Work out the finished part from the listing and answer in its coordinate system (mm). A direction names the side the tool comes from. Give positions to 0.01 mm unless a question says otherwise; leave off trailing zeros. Order: outer loops, then holes, each group sorted by start corner. A loop starts at its lowest first (then second) coordinate and runs counter-clockwise, first axis right, second up.
```python
from build123d import *

# Parameters (mm, degrees)
EXTRUDE1_DEPTH     = 30
SKETCH3_R          = 1.5
CUT_EXTRUDE1_DEPTH = 30


with BuildPart() as part:
    # Sketch2 → Extrude1 (new body)
    with BuildSketch(Plane.XZ.offset(470)):
        Polygon((-380.315803698, -350.2), (-400.415803698, -350.2), (-400.415803698, -355.15), (-380.315803698, -355.15), (-380.315803698, -375.25), (-400.415803698, -375.25), (-400.415803698, -380.2), (-380.315803698, -380.2), (-375.365803698, -380.2), (-375.365803698, -350.2), align=None)
    extrude(amount=-EXTRUDE1_DEPTH)

    # Sketch3 → Cut-Extrude1 (cut)
    with BuildSketch(Plane.XY.offset(-350.2)):
        with Locations((-384.365803698, -465)):
            Circle(SKETCH3_R)
        with Locations((-396.365803698, -465)):
            Circle(SKETCH3_R)
        with Locations((-384.365803698, -450)):
            Circle(SKETCH3_R)
        with Locations((-396.365803698, -450)):
            Circle(SKETCH3_R)
    extrude(amount=-CUT_EXTRUDE1_DEPTH, mode=Mode.SUBTRACT)


solid = part.part
```
1. The part is cut by section C-C (x = -396.25). Write down the section's boundary in (y, z), then the cut area to 3 significant figures.
Findings below:
outline: (-470, -380.2) - (-466.5, -380.2) - (-466.5, -375.25) - (-470, -375.25) - close; (-470, -355.15) - (-466.5, -355.15) - (-466.5, -350.2) - (-470, -350.2) - close; (-463.5, -380.2) - (-451.5, -380.2) - (-451.5, -375.25) - (-463.5, -375.25) - close; (-463.5, -355.15) - (-451.5, -355.15) - (-451.5, -350.2) - (-463.5, -350.2) - close; (-448.5, -380.2) - (-440, -380.2) - (-440, -375.25) - (-448.5, -375.25) - close; (-448.5, -355.15) - (-440, -355.15) - (-440, -350.2) - (-448.5, -350.2) - close
area: 238 mm2
2. The part is cut by section D-D (z = -370.75). Write down the section's boundary in (x, y).
Findings below:
outline: (-380.32, -470) - (-375.37, -470) - (-375.37, -440) - (-380.32, -440) - close
3. The part is cut by section B-B (x = -391). Write down the section's boundary in (y, z).
Findings below:
outline: (-470, -380.2) - (-440, -380.2) - (-440, -375.25) - (-470, -375.25) - close; (-470, -355.15) - (-440, -355.15) - (-440, -350.2) - (-470, -350.2) - close
4. Straight lines are drawn through the part: probe 1 along X at (y, z) = (-465, -378.7); probe 2 along Z at (x, y) = (-384.5, -454.25); probe 3 along Y at (x, z) = (-383.75, -353). For each, find the intervals that lie inside material, in ascending order.
Findings below:
probe 1: x = -400.42 to -397.87, -394.87 to -385.87, -382.87 to -375.37
probe 2: z = -380.2 to -375.25, -355.15 to -350.2
probe 3: y = -470 to -466.37, -463.63 to -451.37, -448.63 to -440
5. The part is cut by section A-A (y = -450). Write down the section's boundary in (x, z), then the cut area to 3 significant figures.
Findings below:
outline: (-400.42, -380.2) - (-397.87, -380.2) - (-397.87, -375.25) - (-400.42, -375.25) - close; (-400.42, -355.15) - (-397.87, -355.15) - (-397.87, -350.2) - (-400.42, -350.2) - close; (-394.87, -380.2) - (-385.87, -380.2) - (-385.87, -375.25) - (-394.87, -375.25) - close; (-394.87, -355.15) - (-385.87, -355.15) - (-385.87, -350.2) - (-394.87, -350.2) - close; (-382.87, -380.2) - (-375.37, -380.2) - (-375.37, -350.2) - (-382.87, -350.2) - (-382.87, -355.15) - (-380.32, -355.15) - (-380.32, -375.25) - (-382.87, -375.25) - close
area: 288 mm2
6. The mould has two halves that part along Y. Classify faces 1 (the face through (-390, -455, -375.25)), 2 (the face through (-380, -470, -362)), 3 (the face through (-383.67, -451.33, -352.64)): pulls with the +Y half, pulls with the -Y half, needs draft (parallel to the pull), parting line crosses it, or undercut.
Findings below:
face 1: needs draft
face 2: pulls with the -Y half
face 3: undercut
7. Which of the six approach directions +Z, -Z, +X, -X, +Y, -Y give full straight-line access (tool end or side, diameter ignored) to faces 4 (the face through (-395.67, -466.33, -352.64)), 5 (the face through (-391, -455, -355.15))?
Findings below:
face 4: +Z, -Z
face 5: -X, +Y, -Y
